Here's how the part is built. I have some questions about the finished solid (model axes, mm). A direction names the side the tool comes from. Round coordinates to 2 decimals unless told otherwise and drop trailing zeros. Loops run counter-clockwise (first coordinate to the right, second up) from the corner with the lowest first, then second, coordinate; pieces in that order, holes last. Notation, with made-up numbers: M -17.5,4.5 L 38.5,4.5 A33 cw 38.5,36.5 Z; hole C 87.5,-35.5 d8. An arc over 180 degrees is marked long. Put each result on its own line as item: value. Start each with the question number.
```python
from build123d import *

# Parameters (mm, degrees)
SKETCH3_R             = 4
BOSS_EXTRUDE1_DEPTH   = 11
BOSS_EXTRUDE1_2_DEPTH = 11
BOSS_EXTRUDE1_3_DEPTH = 11
BOSS_EXTRUDE1_4_DEPTH = 11
SKETCH6_R             = 7.5
BOSS_EXTRUDE6_DEPTH   = 8
SKETCH8_R             = 1.6
CUT_EXTRUDE1_DEPTH    = 35.190934471
SKETCH9_R             = 3
CUT_EXTRUDE2_DEPTH    = 3
BOSS_EXTRUDE8_START   = -11
SKETCH10_R            = 4.1
SKETCH10_R_2          = 4
BOSS_EXTRUDE8_DEPTH   = 11
SKETCH11_R            = 2.7
SKETCH11_R_2          = 2.15
CUT_EXTRUDE3_DEPTH    = 8
BOSS_EXTRUDE9_START   = -4
SKETCH12_R            = 7.5
SKETCH12_R_2          = 7
BOSS_EXTRUDE9_DEPTH   = 4
CHAMFER1_SIZE         = 0.5


with BuildPart() as part:
    # Sketch3 → Boss-Extrude1 (new body)
    with BuildSketch(Plane(origin=(0, 0, -116.757942017), x_dir=(-1, 0, 0), z_dir=(0, 0, -1))):
        with Locations((-11.66726189, 11.66726189)):
            Circle(SKETCH3_R)
    extrude(amount=BOSS_EXTRUDE1_DEPTH)



with BuildPart() as body_2:
    # Sketch3 → Boss-Extrude1 2 (new body)
    with BuildSketch(Plane(origin=(0, 0, -116.757942017), x_dir=(-1, 0, 0), z_dir=(0, 0, -1))):
        with Locations((11.66726189, 11.66726189)):
            Circle(SKETCH3_R)
    extrude(amount=BOSS_EXTRUDE1_2_DEPTH)


with BuildPart() as body_3:
    # Sketch3 → Boss-Extrude1 3 (new body)
    with BuildSketch(Plane(origin=(0, 0, -116.757942017), x_dir=(-1, 0, 0), z_dir=(0, 0, -1))):
        with Locations((11.66726189, -11.66726189)):
            Circle(SKETCH3_R)
    extrude(amount=BOSS_EXTRUDE1_3_DEPTH)


with BuildPart() as body_4:
    # Sketch3 → Boss-Extrude1 4 (new body)
    with BuildSketch(Plane(origin=(0, 0, -116.757942017), x_dir=(-1, 0, 0), z_dir=(0, 0, -1))):
        with Locations((-11.66726189, -11.66726189)):
            Circle(SKETCH3_R)
    extrude(amount=BOSS_EXTRUDE1_4_DEPTH)


with BuildPart() as part_1:
    add(part.part)

    add(body_2.part)  # Boss-Extrude6 merges body 2

    add(body_3.part)  # Boss-Extrude6 merges body 3

    add(body_4.part)  # Boss-Extrude6 merges body 4
    # Sketch6 → Boss-Extrude6 (add)
    with BuildSketch(Plane.XY.offset(-116.757942017)):
        with BuildLine():
            ThreePointArc((16.992766074, -10.735730117), (19.607007689, 4.424392555), (10.735730117, 16.992766074))
            ThreePointArc((10.735730117, 16.992766074), (-4.424392555, 19.607007689), (-16.992766074, 10.735730117))
            ThreePointArc((-16.992766074, 10.735730117), (-19.607007689, -4.424392555), (-10.735730117, -16.992766074))
            ThreePointArc((-10.735730117, -16.992766074), (4.424392555, -19.607007689), (16.992766074, -10.735730117))
        make_face()
        Circle(SKETCH6_R, mode=Mode.SUBTRACT)
    extrude(amount=BOSS_EXTRUDE6_DEPTH)

    # Sketch8 → Cut-Extrude1 (cut, through all)
    with BuildSketch(Plane.XY.offset(-108.757942017)):
        with Locations((11.66726189, 11.66726189)):
            Circle(SKETCH8_R)
        with Locations((11.66726189, -11.66726189)):
            Circle(SKETCH8_R)
        with Locations((-11.66726189, -11.66726189)):
            Circle(SKETCH8_R)
        with Locations((-11.66726189, 11.66726189)):
            Circle(SKETCH8_R)
    extrude(amount=-CUT_EXTRUDE1_DEPTH, mode=Mode.SUBTRACT)

    # Sketch9 → Cut-Extrude2 (cut)
    with BuildSketch(Plane.XY.offset(-127.757942017)):
        with Locations(Location((11.66726189, 11.66726189, 0), (0, 0, 180))):
            Circle(SKETCH9_R)
        with Locations(Location((11.66726189, -11.66726189, 0), (0, 0, 180))):
            Circle(SKETCH9_R)
        with Locations(Location((-11.66726189, -11.66726189, 0), (0, 0, 180))):
            Circle(SKETCH9_R)
        with Locations(Location((-11.66726189, 11.66726189, 0), (0, 0, 180))):
            Circle(SKETCH9_R)
    extrude(amount=CUT_EXTRUDE2_DEPTH, mode=Mode.SUBTRACT)

    # Sketch10 → Boss-Extrude8 (add)
    # profile 1 of 4: a face of its own
    with BuildSketch(Plane(origin=(0, 0, -127.757942017), x_dir=(-1, 0, 0), z_dir=(0, 0, -1)).offset(BOSS_EXTRUDE8_START)):
        with Locations((11.66726189, 11.66726189)):
            Circle(SKETCH10_R)
        with Locations((11.66726189, 11.66726189)):
            Circle(SKETCH10_R_2, mode=Mode.SUBTRACT)
    # profile 2 of 4: a face of its own
    with BuildSketch(Plane(origin=(0, 0, -127.757942017), x_dir=(-1, 0, 0), z_dir=(0, 0, -1)).offset(BOSS_EXTRUDE8_START)):
        with Locations((11.66726189, -11.66726189)):
            Circle(SKETCH10_R)
        with Locations((11.66726189, -11.66726189)):
            Circle(SKETCH10_R_2, mode=Mode.SUBTRACT)
    # profile 3 of 4: a face of its own
    with BuildSketch(Plane(origin=(0, 0, -127.757942017), x_dir=(-1, 0, 0), z_dir=(0, 0, -1)).offset(BOSS_EXTRUDE8_START)):
        with Locations((-11.66726189, -11.66726189)):
            Circle(SKETCH10_R)
        with Locations((-11.66726189, -11.66726189)):
            Circle(SKETCH10_R_2, mode=Mode.SUBTRACT)
    # profile 4 of 4: a face of its own
    with BuildSketch(Plane(origin=(0, 0, -127.757942017), x_dir=(-1, 0, 0), z_dir=(0, 0, -1)).offset(BOSS_EXTRUDE8_START)):
        with Locations((-11.66726189, 11.66726189)):
            Circle(SKETCH10_R)
        with Locations((-11.66726189, 11.66726189)):
            Circle(SKETCH10_R_2, mode=Mode.SUBTRACT)
    extrude(amount=BOSS_EXTRUDE8_DEPTH)

    # Sketch11 → Cut-Extrude3 (cut)
    with BuildSketch(Plane.XY.offset(-108.757942017)):
        with Locations((0, 15)):
            Circle(SKETCH11_R)
        with Locations((15, 0)):
            Circle(SKETCH11_R)
        with Locations((0, -15)):
            Circle(SKETCH11_R)
        with Locations((-15, 0)):
            Circle(SKETCH11_R)
        with Locations((-11.66726189, 11.66726189)):
            Circle(SKETCH11_R_2)
        with Locations((11.66726189, 11.66726189)):
            Circle(SKETCH11_R_2)
        with Locations((11.66726189, -11.66726189)):
            Circle(SKETCH11_R_2)
        with Locations((-11.66726189, -11.66726189)):
            Circle(SKETCH11_R_2)
    extrude(amount=-CUT_EXTRUDE3_DEPTH, mode=Mode.SUBTRACT)

    # Sketch12 → Boss-Extrude9 (add)
    with BuildSketch(Plane.XY.offset(-108.757942017).offset(BOSS_EXTRUDE9_START)):
        Circle(SKETCH12_R)
        Circle(SKETCH12_R_2, mode=Mode.SUBTRACT)
    extrude(amount=BOSS_EXTRUDE9_DEPTH)

    # Chamfer1
    chamfer1_edges = [part_1.edges().sort_by_distance(p)[0] for p in [
        (-10.735730117, -16.992766074, -108.757942017),
        (-7, 0, -108.757942017),
    ]]
    chamfer(chamfer1_edges, length=CHAMFER1_SIZE)


solid = part_1.part
```
1) On a 3-axis mill with a long thin cutter (end or side, diameter ignored), from which of +Z, -Z, +X, -X, +Y, -Y can I reach the whole of each face in a straight line? I mean faces 1 (the face through (-0.351, 17.677, -112.702)), 2 (the face through (-13.815, -11.573, -112.702)), 3 (the face through (-13.052, -9.006, -126.279)). Say none if no direction works.
2) If we mould it in two halves opening along X, with no side actions, what happens to faces 4 (the face through (17.575, 0.811, -112.702)), 5 (the face through (11, -15, -127.758))? For each: pulls with the +X half, pulls with the -X half, needs draft (parallel to the pull), parting line crosses it, or undercut.
3) Suppose I cut it at C-C (z = -111.5). State how many separate pieces and enclosed holes the cut face has, plus the area to 3 significant figures.
4) Suppose I cut it at B-B (x = 0). Write out the boundary of the cut face in (y, z), plus the area to 3 significant figures.
5) If I drill on probe 1 along Y at (x, z) = (-13.5, -114.75) (3 decimals); probe 2 along X at (y, z) = (-1, -110.25); probe 3 along Z at (x, y) = (-17.5, 3), over which ranges is the centre line in solid material (lowest first)? Write a range as from..to.
6) I'm going to push flat-ended pins straight in: P1, Ø4, axis at x = 11.67, y = -11.67, coming from the -Z side; P2, Ø9.5, axis at x = 11.67, y = 11.67, coming from the +Z side; P3, Ø1.5, axis at x = 13.5, z = -120.5, coming from the +Y side; P4, Ø2, axis at x = -12.5, z = -117, coming from the -Y side. Where does each tip first touch, or does it pass through?
7) Suppose I cut it at A-A (z = -120). Write out the boundary of the cut face in (x, y), plus the area to 3 significant figures.
8) Suppose I cut it at D-D (z = -126.5). Write out the boundary of the cut face in (x, y).
Results are:
1. face 1: +Z, -Z
1. face 2: +Z
1. face 3: -Z
2. face 4: undercut
2. face 5: needs draft
3. separate pieces: 1
3. enclosed holes: 9
3. area: 966 mm²
4. outline: M -20.1,-116.76 L -17.7,-116.76 L -17.7,-108.76 L -19.6,-108.76 L -20.1,-109.26 Z; M -12.3,-116.76 L -7.5,-116.76 L -7.5,-112.76 L -7,-112.76 L -7,-109.26 L -7.5,-108.76 L -12.3,-108.76 Z; M 7,-112.76 L 7.5,-112.76 L 7.5,-116.76 L 12.3,-116.76 L 12.3,-108.76 L 7.5,-108.76 L 7,-109.26 Z; M 17.7,-116.76 L 20.1,-116.76 L 20.1,-109.26 L 19.6,-108.76 L 17.7,-108.76 Z
4. area: 119 mm²
5. probe 1: -14.892..-12.791, -10.543..-2.245, 2.245..10.543, 12.791..14.892
5. probe 2: -20.08..-17.51, -12.49..-6.93, 6.93..12.49, 17.51..20.08
5. probe 3: -116.76..-108.76
6. P1: z = -124.76
6. P2: z = -108.76
6. P3: y = 15.62
6. P4: y = -16.46
7. outline: C -11.67,-11.67 d8.2; C -11.67,11.67 d8.2; C 11.67,-11.67 d8.2; C 11.67,11.67 d8.2; hole C -11.67,-11.67 d3.2; hole C -11.67,11.67 d3.2; hole C 11.67,-11.67 d3.2; hole C 11.67,11.67 d3.2
7. area: 179 mm²
8. outline: C -11.67,-11.67 d8.2; C -11.67,11.67 d8.2; C 11.67,-11.67 d8.2; C 11.67,11.67 d8.2; hole C -11.67,-11.67 d6; hole C -11.67,11.67 d6; hole C 11.67,-11.67 d6; hole C 11.67,11.67 d6
